Part model, mm, in its own coordinate system. A direction names the side the tool comes from. Round coordinates to 2 decimals unless told otherwise and drop trailing zeros. Write each loop counter-clockwise with the first axis right and the second up, starting at its lowest first coordinate (ties: lowest second). Pieces come first, ordered by that corner, then holes. Notation, with made-up numbers: M 5,11.5 L 47,11.5 A20 ccw 47,30.5 Z; hole C 65.25,89 d3. An arc over 180 degrees is marked long. Answer as a JSON object with one key per item and string values. Group by question number.
1. Two-plate mould, pull along Z, no slides. Class faces 4 (the face through (6.946, -3.604, -11.87)), 5 (the face through (8, 0, 4)), 6 (the face through (-5, 0, 3.5)): +Z half, -Z half, draft (parallel to the pull), parting line (faces both ways), or undercut.
2. Drill centre lines: line 1 (Z direction, x = 4, y = -10); line 2 (X direction, y = -0.5, z = -0.75); line 3 (Z direction, x = 5.5, y = -7). Where is each one in solid material? Low to high. Write a range as from..to.
3. Drop flat-ended pins along their axis: pin 1 (1 mm diameter, centred on x = -4.5, z = -16.5, fed in from +Y); pin 2 (5 mm diameter, centred on x = 4, y = -4, fed in from +Z); pin 3 (1.6 mm diameter, centred on y = 7, z = 4, fed in from -X). Give the stop position or say it passes through.
4. Band-saw the part on C-C, the plane x = 12. Write the cut outline in (y, z), plus the area to 3 significant figures.
5. Band-saw the part on D-D, the plane z = -4.75. Write the cut outline in (x, y).
6. Band-saw the part on A-A, the plane z = 0. Write the cut outline in (x, y).
7. Which spindle directions (+Z, -Z, +X, -X, +Y, -Y) get a long thin tool onto all of the face, cutting with end or side? Do faces 1 (the face through (-11.04, -10.24, -12.25)), 2 (the face through (-17, 0, 0)), 3 (the face through (-15, 12.5, 0)). Say none if no direction does.
from build123d import *

# Parameters (mm, degrees)
SKETCH1_W           = 34
SKETCH1_H           = 29
BOSS_EXTRUDE1_DEPTH = 3.5
SKETCH2_W           = 9
SKETCH2_H           = 29
BOSS_EXTRUDE2_DEPTH = 2
CUT_EXTRUDE1_DEPTH  = 25.088378941
SKETCH5_R           = 9.75
CUT_EXTRUDE2_DEPTH  = 5
CUT_EXTRUDE2_DRAFT  = -45


with BuildPart() as part:
    # Sketch1 → Boss-Extrude1 (new, symmetric)
    with BuildSketch(Plane.XY):
        Rectangle(SKETCH1_W, SKETCH1_H)
    extrude(amount=BOSS_EXTRUDE1_DEPTH, both=True)

    # Sketch2 → Boss-Extrude2 (add)
    with BuildSketch(Plane.XY.offset(3.5)):
        with Locations((12.5, 0)):
            Rectangle(SKETCH2_W, SKETCH2_H)
    extrude(amount=BOSS_EXTRUDE2_DEPTH)

    # Sketch3 → Cut-Extrude1 (cut, through all)
    with BuildSketch(Plane(origin=(0, 0, -3.5), x_dir=(-1, 0, 0), z_dir=(0, 0, -1))):
        Polygon((-14, -14.5), (-17, -9.5), (-17, -14.5), align=None)
        Polygon((13, -14.5), (17, -10.5), (17, -14.5), align=None)
        Polygon((17, 10.5), (13, 14.5), (17, 14.5), align=None)
        Polygon((-17, 9.5), (-14, 14.5), (-17, 14.5), align=None)
    extrude(amount=-CUT_EXTRUDE1_DEPTH, mode=Mode.SUBTRACT)

    # Sketch4 → Revolve1 (revolve)
    with BuildSketch(Plane(origin=(0, 0, 0), x_dir=(1, 0, 0), z_dir=(0, 1, 0)), mode=Mode.PRIVATE) as revolve1_sk:
        Polygon((-17, 3.5), (-4.5, 3.5), (-4.5, 24.25), (-18.25, 24.25), (-18.25, 22.25), (-17, 22.25), (-17, 20.25), (-18.25, 20.25), (-18.25, 19.25), (-17, 19.25), (-17, 12.25), (-16.5, 12.25), (-16.5, 11.5), (-17, 11.5), align=None)
    revolve(revolve1_sk.sketch.rotate(Axis((-4.5, 0, -3.5), (0, 0, -1)), 180), axis=Axis((-4.5, 0, -3.5), (0, 0, -1)))


with BuildPart() as cut_extrude2_tool:
    # Sketch5 → Cut-Extrude2 (with draft: the straight prism first)
    with BuildSketch(Plane(origin=(0, 0, -24.25), x_dir=(-1, 0, 0), z_dir=(0, 0, -1))):
        with Locations((4.5, 0)):
            Circle(SKETCH5_R)
    extrude(amount=-CUT_EXTRUDE2_DEPTH)
    # Cut-Extrude2: the draft: its side faces are tilted about the plane it starts from
    cut_extrude2_sides = [cut_extrude2_tool.faces().sort_by_distance(p)[0] for p in [
        (5.25, 0, -21.75),
    ]]
    draft(cut_extrude2_sides, Plane(origin=(0, 0, -24.25), x_dir=(-1, 0, 0), z_dir=(0, 0, -1)), CUT_EXTRUDE2_DRAFT)


with BuildPart() as part_1:
    add(part.part)

    # Cut-Extrude2: cut by cut_extrude2_tool
    add(cut_extrude2_tool.part, mode=Mode.SUBTRACT)

    # Sketch6 → Revolve2 (revolve)
    with BuildSketch(Plane(origin=(0, 0, 0), x_dir=(1, 0, 0), z_dir=(0, 1, 0))):
        with BuildLine():
            Line((-9.25, 19.25), (-4.5, 19.25))
            Line((-4.5, 19.25), (-4.5, 24))
            ThreePointArc((-4.5, 24), (-7.858757211, 22.608757211), (-9.25, 19.25))
        make_face()
    revolve(axis=Axis((-4.5, 0, -19.25), (0, 0, -1)))


solid = part_1.part
Worked answers:
{
 "1": {"face 4": "undercut", "face 5": "draft", "face 6": "+Z half"},
 "2": {"line 1": "z = -24.25..-22.25, -20.25..-19.25, -3.5..3.5", "line 2": "x = -17..17", "line 3": "z = -24.25..-12.25, -11.5..3.5"},
 "3": {"pin 1": "stops at y = 12.5", "pin 2": "stops at z = 3.5", "pin 3": "stops at x = -17"},
 "4": {"outline": "M -14.5,-3.5 L 14.5,-3.5 L 14.5,5.5 L -14.5,5.5 Z", "area": "261 mm^2"},
 "5": {"outline": "C -4.5,0 d25"},
 "6": {"outline": "M -17,-10.5 L -13,-14.5 L 14,-14.5 L 17,-9.5 L 17,9.5 L 14,14.5 L -13,14.5 L -17,10.5 Z"},
 "7": {"face 1": "none", "face 2": "+Z, -X, +Y, -Y", "face 3": "+Z, -Z, -X, +Y"}
}
